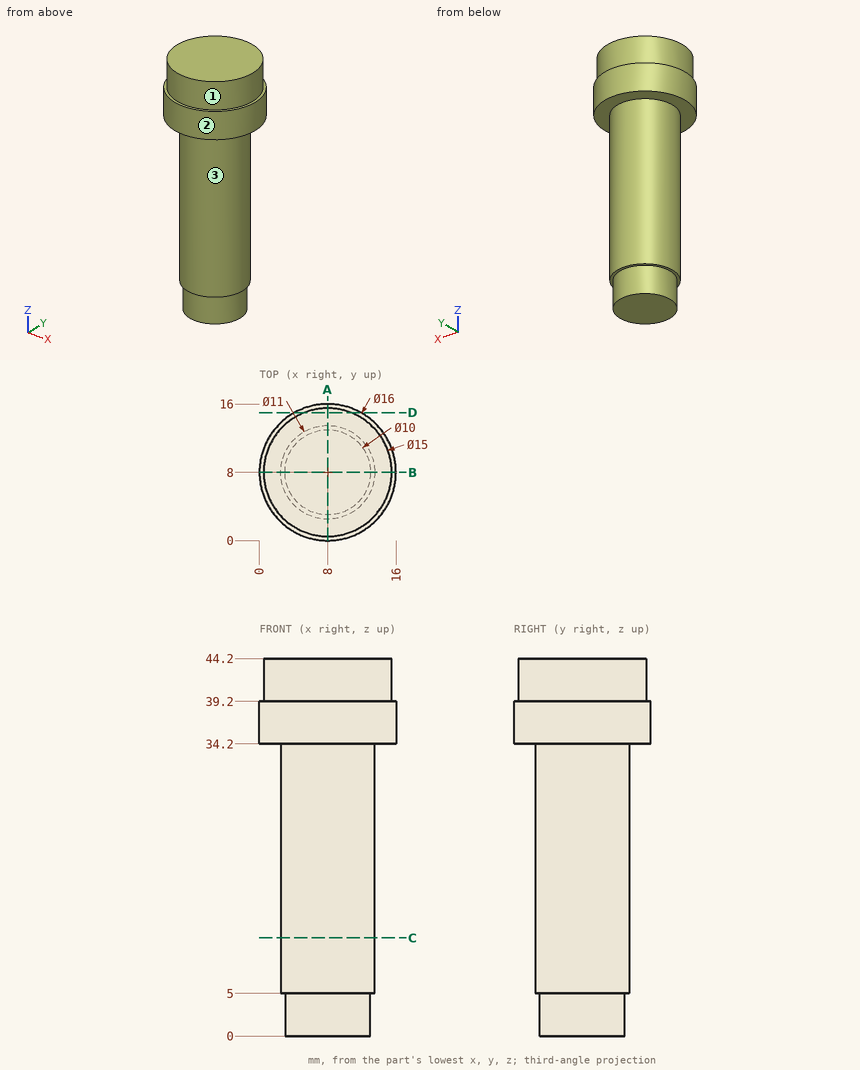
Job drawing, mm, ordinate dimensions from the low corner. One solid piece. A direction names the side the tool comes from. Give positions to 0.01 mm unless a question says otherwise; leave off trailing zeros. Loops run counter-clockwise (first coordinate to the right, second up) from the corner with the lowest first, then second, coordinate; pieces in that order, holes last. Notation, with made-up numbers: (-39, -23.5) -> (-15, -23.5) arc R28 cw to (-15, -3.5) -> close; hole circle Ø8 at (16.25, 21). An arc over 180 degrees is marked (long way). Use a Markdown table: item, result. Add a question column.
(1) Slice it at C-C on z = 11.5. List the corners of the cut face in (x, y).
(2) Slice it at D-D on y = 15. List the corners of the cut face in (x, z), and give its area (3 significant figures).
(3) Drop flat-ended pins along their axis: pin 1 Ø5 at (y, z) = (4.5, 10) entering from -X; pin 2 Ø4 at (y, z) = (10, 32) entering from -X; pin 3 Ø2 at (x, z) = (9.5, 16.5) entering from -Y. Give the stop position or say it passes through.
(4) Slice it at A-A on x = 8. List the corners of the cut face in (y, z).
(5) Tool access for the marked faces 1, 2 and 3: list every direction of +Z, -Z, +X, -X, +Y, -Y with a clear straight run to the whole face (end or side of a thin tool).
(6) Wall check: line 1 along Z through (x, y) = (11.25, 13.25); line 2 along X through (y, z) = (8, 11); line 3 along Z through (x, y) = (1.5, 12). Give the ranges that are in metal, low to high.
Filled sheet:
| question | item | result |
|---|---|---|
| 1 | outline | circle Ø11 at (8, 8) |
| 2 | outline | (4.13, 34.2) -> (11.87, 34.2) -> (11.87, 39.2) -> (10.69, 39.2) -> (10.69, 44.2) -> (5.31, 44.2) -> (5.31, 39.2) -> (4.13, 39.2) -> close |
| 2 | area | 65.7 mm2 |
| 3 | pin 1 | x = 2.59 |
| 3 | pin 2 | x = 2.5 |
| 3 | pin 3 | y = 2.52 |
| 4 | outline | (0, 34.2) -> (2.5, 34.2) -> (2.5, 5) -> (3, 5) -> (3, 0) -> (13, 0) -> (13, 5) -> (13.5, 5) -> (13.5, 34.2) -> (16, 34.2) -> (16, 39.2) -> (15.5, 39.2) -> (15.5, 44.2) -> (0.5, 44.2) -> (0.5, 39.2) -> (0, 39.2) -> close |
| 5 | face 1 | +Z |
| 5 | face 2 | +Z, -Z |
| 5 | face 3 | -Z |
| 6 | line 1 | 34.2 to 44.2 |
| 6 | line 2 | 2.5 to 13.5 |
| 6 | line 3 | 34.2 to 39.2 |
